The figure shows three views and two pictorial views of one solid part (mm, origin at its lowest corner). Answer the questions. A direction names the side the tool comes from. Round coordinates to 2 decimals unless told otherwise and drop trailing zeros. Order: outer loops, then holes, each group sorted by start corner. A loop starts at its lowest first (then second) coordinate and runs counter-clockwise, first axis right, second up. Notation, with made-up numbers: (-37, 17) -> (-21, 17) arc R24 ccw to (-21, 35) -> close; hole circle Ø9 at (79.25, 79.5). An arc over 180 degrees is marked (long way). Answer as a JSON object with one key per item and string values. Group by question number.
Item 1: Section B-B, the plane z = 8 is taken. Write down the section's boundary in (x, y), plus the area to 3 significant figures.
Item 2: Section C-C, the plane x = 19 is taken. Write down the section's boundary in (y, z), plus the area to 3 significant figures.
Item 3: Section A-A, the plane z = 5 is taken. Write down the section's boundary in (x, y).
Item 4: For the marked faces 1, 2 and 3, determine the directions among +Z, -Z, +X, -X, +Y, -Y from which every point of the face is accessible in a straight line to the end or side of a thin tool.
Item 5: Given P1, Ø0.5, axis at y = 13.5, z = 1.5, coming from the +X side; P2, Ø1.5, axis at y = 9, z = 9, coming from the -X side; P3, Ø1.9, axis at y = 1, z = 1, coming from the +X side, each flat-ended and moving along its own axis, determine where each tip first touches the part or whether it passes through.
Item 6: Consider probe 1 along Z at (x, y) = (5, 5.75); probe 2 along X at (y, z) = (2, 4.25); probe 3 along X at (y, z) = (2.5, 5.75). Determine where each line is inside the solid, lowest interval first. Write a range as from..to.
Item 7: The mould has two halves that part along X. Classify the marked faces 4, 5 and 6: pulls with the +X half, pulls with the -X half, needs draft (parallel to the pull), parting line crosses it, or undercut.
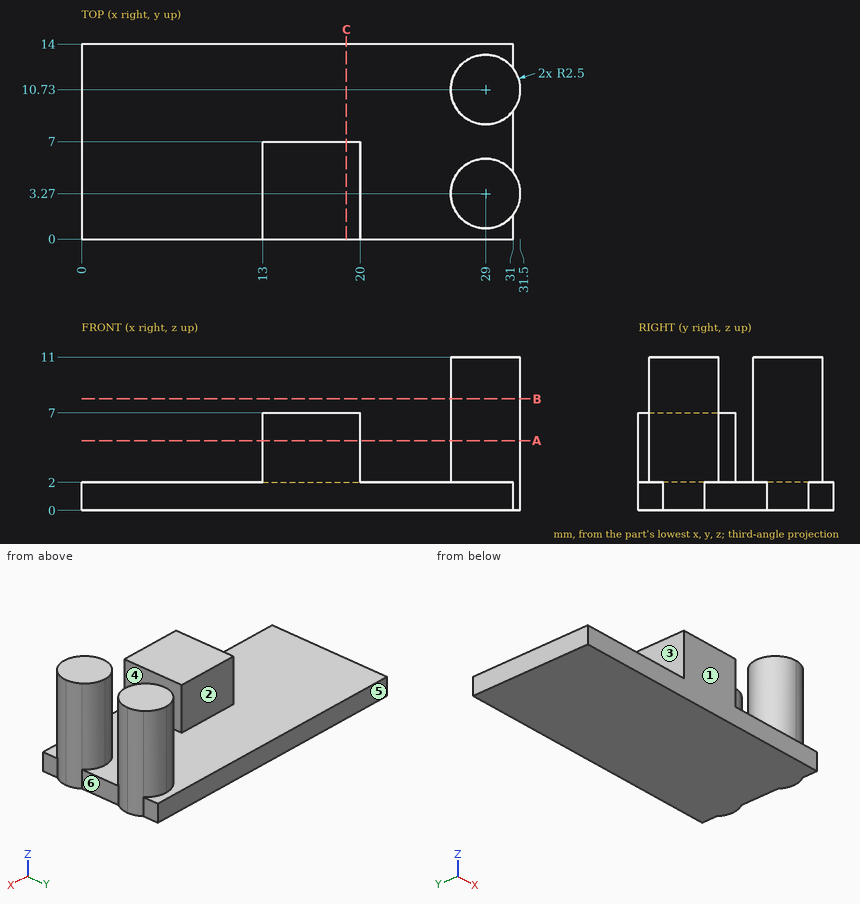
Values found:
{
 "1": {"outline": "circle Ø5 at (29, 3.27); circle Ø5 at (29, 10.73)", "area": "39.3 mm2"},
 "2": {"outline": "(0, 0) -> (14, 0) -> (14, 2) -> (7, 2) -> (7, 7) -> (0, 7) -> close", "area": "63.0 mm2"},
 "3": {"outline": "(13, 0) -> (20, 0) -> (20, 7) -> (13, 7) -> close; circle Ø5 at (29, 3.27); circle Ø5 at (29, 10.73)"},
 "4": {"face 1": "+Z, -Z, +X, -X, -Y", "face 2": "+Z, +X, -X, +Y", "face 3": "+Z, -X, +Y, -Y"},
 "5": {"P1": "x = 31", "P2": "x = 26.7", "P3": "x = 31.12"},
 "6": {"probe 1": "0..2", "probe 2": "13..20, 26.85..31.15", "probe 3": "13..20, 26.62..31.38"},
 "7": {"face 4": "undercut", "face 5": "needs draft", "face 6": "pulls with the +X half"}
}
